Input: dimensioned drawing with shaded views. Units: mm. Origin: part minimum x, y, z. Coordinates: 2 decimals unless noted, no trailing zeros. Order: outer loops, then holes, each group sorted by start corner. A loop starts at its lowest first (then second) coordinate and runs counter-clockwise, first axis right, second up.
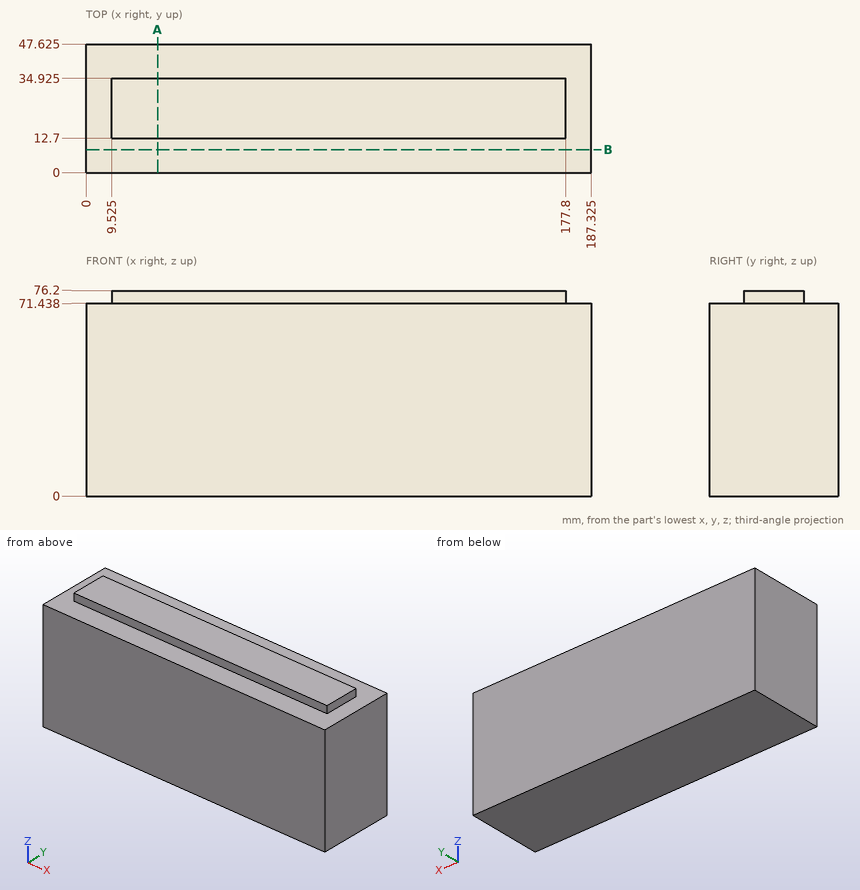
1. Section query B-B on y = 8.5. Return loops of the section in (x, z) (1 decimal), plus the area to 3 significant figures.
Findings:
outline: (0, 0) - (187.3, 0) - (187.3, 71.4) - (0, 71.4) - close
area: 13,400 mm2
2. Ray query, line 1 (Z direction, x = 12.5, y = 36). Return the intervals inside material, ascending.
Findings:
line 1: z = 0 to 71.44
3. Section query A-A on x = 26.5. Return loops of the section in (y, z) (1 decimal).
Findings:
outline: (0, 0) - (47.6, 0) - (47.6, 71.4) - (34.9, 71.4) - (34.9, 76.2) - (12.7, 76.2) - (12.7, 71.4) - (0, 71.4) - close
4. Pin query (flat end, axial travel): P1, Ø6, axis at x = 28.5, y = 31.5, coming from the -Z side; P2, Ø2.5, axis at x = 131, z = 74, coming from the -Y side; P3, Ø2.5, axis at y = 23.5, z = 73.5, coming from the -X side (1 decimal); P4, Ø4, axis at x = 71, z = 74.5, coming from the +Y side (1 decimal). Return the tip coordinate at first contact, or that it passes through.
Findings:
P1: stops at z = 0
P2: stops at y = 12.7
P3: stops at x = 9.5
P4: stops at y = 34.9
